Geometry check sheet. Reference: the model listing, model coordinates, mm. Face numbers are marked on the shaded views. Coordinates: 2 decimals unless noted, no trailing zeros. Write each loop counter-clockwise with the first axis right and the second up, starting at its lowest first coordinate (ties: lowest second). Pieces come first, ordered by that corner, then holes. Notation, with made-up numbers: (84.5, -30.75) -> (106.5, -30.75) arc R24 ccw to (106.5, -12.75) -> close; hole circle Ø2 at (-24, 20). An arc over 180 degrees is marked (long way). Answer in a Markdown table with one row per item. Add a question column.
1. Scan lines: L1, parallel to X at y = 0, z = 8.75; L2, parallel to Y at x = 0, z = 1.75; L3, parallel to X at y = -9.5, z = 14.25. Record each from-to range of solid material in increasing order. Write a range as from..to.
2. Cross-section at B-B on x = 0. Record the cut outline in (y, z).
3. Cross-section at C-C on y = 15.5. Record the cut outline in (x, z).
4. Depth check by flat-ended pin: P1, Ø1, axis at x = -13, z = 2, coming from the -Y side; P2, Ø12, axis at x = 1.5, y = -15.5, coming from the -Z side; P3, Ø2.5, axis at x = 2, y = -22.5, coming from the +Z side; P4, Ø1.7, axis at y = -21.5, z = 12.5, coming from the +X side. Enter the tip coordinate at first touch or a pass-through.
5. Cross-section at D-D on x = -12.5. Record the cut outline in (y, z), and give its area (3 significant figures).
6. Cross-section at A-A on y = 0. Record the cut outline in (x, z), and give its area (3 significant figures).
7. Mould release check, pull along Y, two halves, no side actions. Record for the marked faces 1, 2, 3 and 4: pulls with the +Y half, pulls with the -Y half, needs draft (parallel to the pull), parting line crosses it, or undercut.
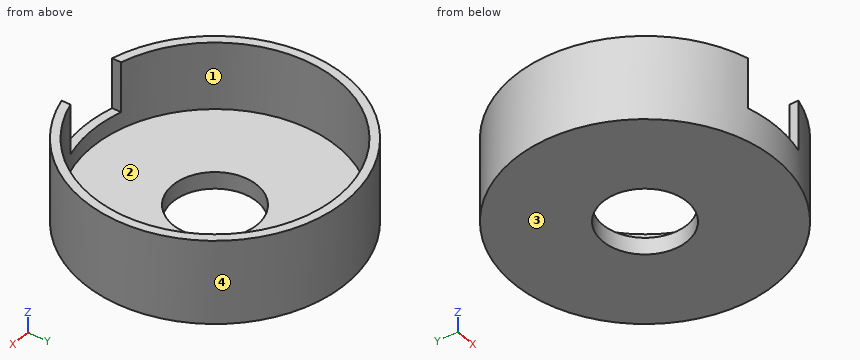
```python
from build123d import *

# Parameters (mm, degrees)
F0_R     = 23.35
F0_R_2   = 21.85
F1_DEPTH = 15
F2_DEPTH = 3
F3_R     = 7.5
F4_DEPTH = 25.4
F6_W     = 12
F6_H     = 6.807694
F7_DEPTH = 9


with BuildPart() as f1:
    # F0 (on Top) → F1 (new body)
    with BuildSketch(Plane.XY):
        Circle(F0_R)
        Circle(F0_R_2, mode=Mode.SUBTRACT)
    extrude(amount=F1_DEPTH)

    # F0 (on Top) → F2 (join)
    with BuildSketch(Plane.XY):
        Circle(F0_R_2)
    extrude(amount=F2_DEPTH)

    # F3 (on Top) → F4 (cut)
    with BuildSketch(Plane.XY):
        Circle(F3_R)
    extrude(amount=F4_DEPTH, mode=Mode.SUBTRACT)

    # F6 (on offset) → F7 (cut)
    with BuildSketch(Plane.XY.offset(15)):
        with Locations((0, -22.193914)):
            Rectangle(F6_W, F6_H)
    extrude(amount=-F7_DEPTH, mode=Mode.SUBTRACT)


solid = f1.part
```
Results found:
| question | item | result |
|---|---|---|
| 1 | L1 | x = -23.35..-21.85, 21.85..23.35 |
| 1 | L2 | y = -23.35..-7.5, 7.5..23.35 |
| 1 | L3 | x = -21.33..-19.68, 19.68..21.33 |
| 2 | outline | (-23.35, 0) -> (-7.5, 0) -> (-7.5, 3) -> (-21.85, 3) -> (-21.85, 6) -> (-23.35, 6) -> close; (7.5, 0) -> (23.35, 0) -> (23.35, 15) -> (21.85, 15) -> (21.85, 3) -> (7.5, 3) -> close |
| 3 | outline | (-17.46, 0) -> (17.46, 0) -> (17.46, 15) -> (15.4, 15) -> (15.4, 3) -> (-15.4, 3) -> (-15.4, 15) -> (-17.46, 15) -> close |
| 4 | P1 | stops at y = -19.72 |
| 4 | P2 | stops at z = 0 |
| 4 | P3 | stops at z = 6 |
| 4 | P4 | stops at x = 10.9 |
| 5 | outline | (-19.72, 0) -> (19.72, 0) -> (19.72, 15) -> (17.92, 15) -> (17.92, 3) -> (-17.92, 3) -> (-17.92, 15) -> (-19.72, 15) -> close |
| 5 | area | 162 mm^2 |
| 6 | outline | (-23.35, 0) -> (-7.5, 0) -> (-7.5, 3) -> (-21.85, 3) -> (-21.85, 15) -> (-23.35, 15) -> close; (7.5, 0) -> (23.35, 0) -> (23.35, 15) -> (21.85, 15) -> (21.85, 3) -> (7.5, 3) -> close |
| 6 | area | 131 mm^2 |
| 7 | face 1 | undercut |
| 7 | face 2 | undercut |
| 7 | face 3 | needs draft |
| 7 | face 4 | parting line crosses it |
